Part print with two shaded views. Sizes in mm from the minimum x, y, z corner. A direction names the side the tool comes from. Coordinates: 2 decimals unless noted, no trailing zeros. Loops run counter-clockwise (first coordinate to the right, second up) from the corner with the lowest first, then second, coordinate; pieces in that order, holes last.
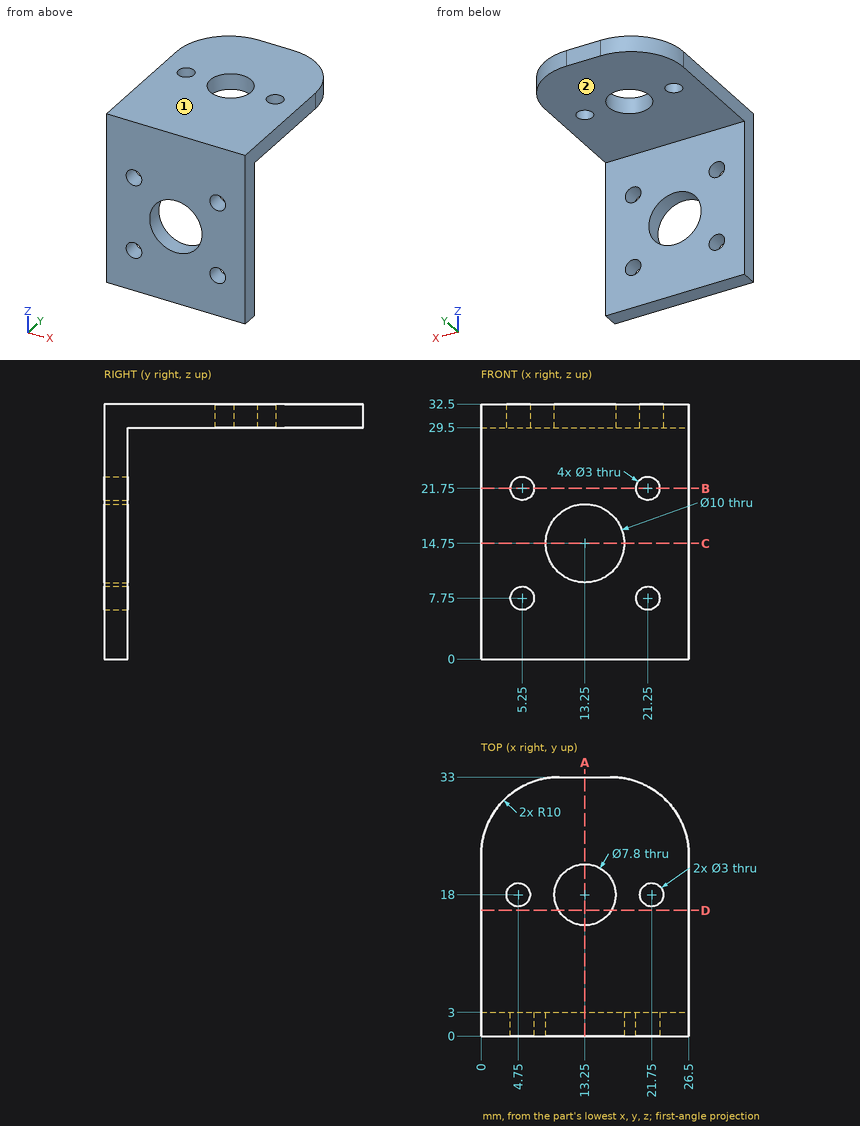
Q1. Slice it at C-C (z = 14.75). List the corners of the cut face in (x, y).
Answers:
outline: (0, 0) - (8.25, 0) - (8.25, 3) - (0, 3) - close; (18.25, 0) - (26.5, 0) - (26.5, 3) - (18.25, 3) - close
Q2. Flat gauge pins, fed straight in: P1, Ø2.5, axis at x = 5.25, z = 7.75, coming from the +Y side; P2, Ø5, axis at x = 20.5, z = 11, coming from the +Y side; P3, Ø2, axis at x = 7.5, y = 11, coming from the -Z side. Where does each tip first touch, or does it go through?
Answers:
P1: passes through
P2: stops at y = 3
P3: stops at z = 29.5
Q3. Slice it at B-B (z = 21.75). List the corners of the cut face in (x, y).
Answers:
outline: (0, 0) - (3.75, 0) - (3.75, 3) - (0, 3) - close; (6.75, 0) - (19.75, 0) - (19.75, 3) - (6.75, 3) - close; (22.75, 0) - (26.5, 0) - (26.5, 3) - (22.75, 3) - close
Q4. Slice it at D-D (y = 16). List the corners of the cut face in (x, z), and give its area (3 significant figures).
Answers:
outline: (0, 29.5) - (9.9, 29.5) - (9.9, 32.5) - (0, 32.5) - close; (16.6, 29.5) - (26.5, 29.5) - (26.5, 32.5) - (16.6, 32.5) - close
area: 59.4 mm2
Q5. Slice it at A-A (x = 13.25). List the corners of the cut face in (y, z).
Answers:
outline: (0, 0) - (3, 0) - (3, 9.75) - (0, 9.75) - close; (0, 19.75) - (3, 19.75) - (3, 29.5) - (14.1, 29.5) - (14.1, 32.5) - (0, 32.5) - close; (21.9, 29.5) - (33, 29.5) - (33, 32.5) - (21.9, 32.5) - close
Q6. Drill centre lines: line 1 (Z direction, x = 5.25, y = 1.55); line 2 (X direction, y = 1.35, z = 7.75); line 3 (Y direction, x = 13.25, z = 30.55). Where is each one in solid material? Low to high.
Answers:
line 1: z = 0 to 6.25, 9.25 to 20.25, 23.25 to 32.5
line 2: x = 0 to 3.75, 6.75 to 19.75, 22.75 to 26.5
line 3: y = 0 to 14.1, 21.9 to 33
Q7. Which spindle directions (+Z, -Z, +X, -X, +Y, -Y) get a long thin tool onto all of the face, cutting with end or side? Do the marked faces 1 and 2. Say none if no direction does.
Answers:
face 1: +Z, +X, -X, +Y, -Y
face 2: -Z, +X, -X, +Y
